from build123d import *

# Parameters (mm, degrees)
F0_W     = 43.8
F0_H     = 43.8
F1_DEPTH = 9
F3_DEPTH = 43.8
F5_DEPTH = 4


with BuildPart() as f1:
    # F0 (on Top) → F1 (new body)
    with BuildSketch(Plane.XY):
        with Locations((6.28503, 0.571359)):
            Rectangle(F0_W, F0_H)
    extrude(amount=F1_DEPTH)

    # F2 (on face) → F3 (cut, through all)
    with BuildSketch(Plane.XZ.offset(21.328641)):
        Polygon((-15.61497, 0), (-11.21497, 9), (-15.61497, 9), align=None)
        Polygon((28.18503, 9), (23.78503, 9), (28.18503, 0), align=None)
    extrude(amount=-F3_DEPTH, mode=Mode.SUBTRACT)

    # F4 (on face) → F5 (cut)
    with BuildSketch(Plane(origin=(0, 0, 0), x_dir=(1, 0, 0), z_dir=(0, 0, -1))):
        with BuildLine():
            ThreePointArc((10.527671, -4.814), (11.828308, -2.86746), (12.28503, -0.571359))
            ThreePointArc((12.28503, -0.571359), (11.828308, 1.724742), (10.527671, 3.671282))
            Line((10.527671, 3.671282), (6.28503, -0.571359))
            Line((6.28503, -0.571359), (10.527671, -4.814))
        make_face()
        with BuildLine():
            Line((6.28503, -0.571359), (10.527671, 3.671282))
            ThreePointArc((10.527671, 3.671282), (6.28503, 5.428641), (2.04239, 3.671282))
            Line((2.04239, 3.671282), (6.28503, -0.571359))
        make_face()
        with BuildLine():
            ThreePointArc((2.04239, -4.814), (6.28503, -6.571359), (10.527671, -4.814))
            Line((10.527671, -4.814), (6.28503, -0.571359))
            Line((6.28503, -0.571359), (2.04239, -4.814))
        make_face()
        with BuildLine():
            Line((6.28503, -0.571359), (2.04239, 3.671282))
            ThreePointArc((2.04239, 3.671282), (0.28503, -0.571359), (2.04239, -4.814))
            Line((2.04239, -4.814), (6.28503, -0.571359))
        make_face()
    extrude(amount=-F5_DEPTH, mode=Mode.SUBTRACT)


solid = f1.part
Verification items for the finished model (mm, model axes). Coordinates: 2 decimals unless noted, no trailing zeros. Order: outer loops, then holes, each group sorted by start corner. A loop starts at its lowest first (then second) coordinate and runs counter-clockwise, first axis right, second up. Notation, with made-up numbers: M -24.5,9.5 L 16.5,9.5 A25 ccw 16.5,31.5 Z; hole C 33,-3 d4. An arc over 180 degrees is marked long. Return JSON: item names as keys, results as strings.
1) Thickness scan on L1, parallel to X at y = -3.5, z = 1; L2, parallel to Z at x = 9, y = 2.5; L3, parallel to X at y = 1, z = 2. Record the ranges inside material, lowest first. Write a range as [from, to].
Answer list:
{"L1": "[-15.13, 1.88], [10.69, 27.7]", "L2": "[4, 9]", "L3": "[-14.64, 0.3], [12.27, 27.21]"}
2) Cross-section at C-C, the plane z = 1. Record the boundary of the cut face in (x, y), and give its area (3 significant figures).
Answer list:
{"outline": "M -15.13,-21.33 L 27.7,-21.33 L 27.7,22.47 L -15.13,22.47 Z; hole M 2.04,-3.67 A6 ccw 10.53,-3.67 A6 ccw 12.29,0.57 A6 ccw 10.53,4.81 A6 ccw 2.04,4.81 A6 ccw Z", "area": "1,760 mm2"}
3) Cross-section at B-B, the plane y = -2. Record the boundary of the cut face in (x, z).
Answer list:
{"outline": "M -15.61,0 L 0.86,0 L 0.86,4 L 11.71,4 L 11.71,0 L 28.19,0 L 23.79,9 L -11.21,9 Z"}
4) Cross-section at A-A, the plane x = 4. Record the boundary of the cut face in (y, z), and give its area (3 significant figures).
Answer list:
{"outline": "M -21.33,0 L -4.98,0 L -4.98,4 L 6.12,4 L 6.12,0 L 22.47,0 L 22.47,9 L -21.33,9 Z", "area": "350 mm2"}
5) Cross-section at D-D, the plane z = 7.5. Record the boundary of the cut face in (x, y), and give its area (3 significant figures).
Answer list:
{"outline": "M -11.95,-21.33 L 24.52,-21.33 L 24.52,22.47 L -11.95,22.47 Z", "area": "1,600 mm2"}
6) Release check for a two-part mould opening along X. For faces 1 (the flat face through (6, 0, 4)), 2 (the flat face through (6, 22.471, 4)), 3 (the flat face through (-13.446, 0.265, 4.437)) record: +X half, -X half, draft (parallel to the pull), parting line (faces both ways), or undercut.
Answer list:
{"face 1": "undercut", "face 2": "draft", "face 3": "-X half"}
7) Gauge pin test, flat ends, axial feed: pin 1 (3 mm diameter, centred on x = 0, y = -12.5, fed in from -Z); pin 2 (2 mm diameter, centred on y = 1.5, z = 5.5, fed in from -X) (3 decimals); pin 3 (6 mm diameter, centred on x = 8, y = 1.5, fed in from -Z). Record the tip position at first contact, or that the pin passes through.
Answer list:
{"pin 1": "z = 0", "pin 2": "x = -13.415", "pin 3": "z = 4"}
